Model file for the job. Use its own axes, mm. Round coordinates to 2 decimals unless told otherwise and drop trailing zeros. Order: outer loops, then holes, each group sorted by start corner. A loop starts at its lowest first (then second) coordinate and runs counter-clockwise, first axis right, second up. Notation, with made-up numbers: (83.5, 30.25) - (137.5, 30.25) arc R20 ccw to (137.5, 57.25) - close; hole circle Ø8 at (10, -1). An arc over 180 degrees is marked (long way). Use one line per item in the form item = value.
from build123d import *

# Parameters (mm, degrees)
ESQUISSE1_R        = 3
BOSS_EXTRU_1_DEPTH = 5


with BuildPart() as part:
    # Esquisse1 → Boss.-Extru.1 (new body)
    with BuildSketch(Plane.XY):
        Polygon((-2.485281374, 6), (-4.242640687, 4.242640687), (-6, 2.485281374), (-6, 0), (-6, -2.485281374), (-4.242640687, -4.242640687), (-2.485281374, -6), (2.485281374, -6), (4.242640687, -4.242640687), (6, -2.485281374), (6, 2.485281374), (4.242640687, 4.242640687), (2.485281374, 6), align=None)
        Circle(ESQUISSE1_R, mode=Mode.SUBTRACT)
    extrude(amount=BOSS_EXTRU_1_DEPTH)


solid = part.part
(1) Pin check, flat tips, straight feed: pin 1 (3.5 mm diameter, centred on x = 0, y = 0, fed in from -Z); pin 2 (1 mm diameter, centred on x = 3.5, z = 3.5, fed in from +Y). Stop position of each tip, or through.
Report:
pin_1 = through
pin_2 = 5.49
(2) Slice it at A-A on x = 0. Give the cut face in (y, z), then the cut area to 3 significant figures.
Report:
outline = (-6, 0) - (-3, 0) - (-3, 5) - (-6, 5) - close; (3, 0) - (6, 0) - (6, 5) - (3, 5) - close
area = 30.0 mm2
(3) Probe probe 1 along Y at (x, z) = (0, 3.25); probe 2 along X at (y, z) = (-0.5, 1.1); probe 3 along Y at (x, z) = (2, 1.3). List the from-to ranges inside material, lowest first. Write a range as [from, to].
Report:
probe_1 = [-6, -3], [3, 6]
probe_2 = [-6, -2.96], [2.96, 6]
probe_3 = [-6, -2.24], [2.24, 6]
(4) Pull direction Y, two halves, no side cores. Call faces 1 (the face through (-3, 0, 2)), 2 (the face through (-6, 0, 2)), 3 (the face through (-4.267, -4.218, 2.465)), 4 (the face through (4.267, 4.218, 2.465)): released by +Y, released by -Y, zero draft, split by the parting line, or undercut.
Report:
face_1 = undercut
face_2 = zero draft
face_3 = released by -Y
face_4 = released by +Y
(5) Slice it at C-C on z = 2.3. Give the cut face in (x, y).
Report:
outline = (-6, -2.49) - (-2.49, -6) - (2.49, -6) - (6, -2.49) - (6, 2.49) - (2.49, 6) - (-2.49, 6) - (-6, 2.49) - close; hole circle Ø6 at (0, 0)
(6) Slice it at D-D on y = 3.5. Give the cut face in (x, z), then the cut area to 3 significant figures.
Report:
outline = (-4.99, 0) - (4.99, 0) - (4.99, 5) - (-4.99, 5) - close
area = 49.9 mm2
